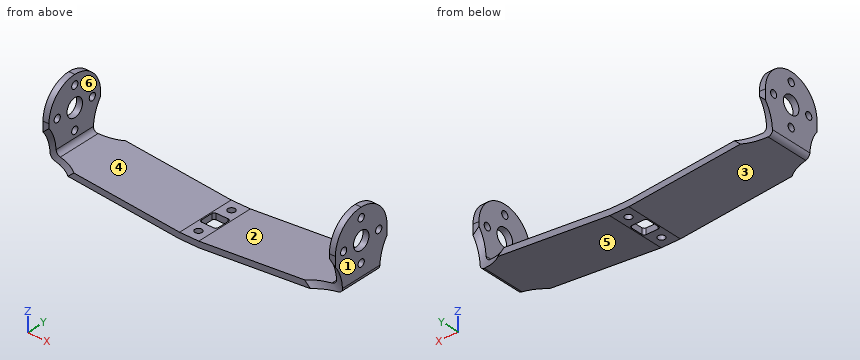
```python
from build123d import *

# Parameters (mm, degrees)
RESSALTO_EXTRUS_O1_DEPTH = 25
FILETE1_R                = 12.5
FILETE2_R                = 2
ESBO_O2_R                = 1.5
CORTE_EXTRUS_O1_DEPTH    = 10
ESBO_O3_R                = 3.75
ESBO_O3_R_2              = 1.5
CORTE_EXTRUS_O2_DEPTH    = 131.832972904
ESBO_O4_R                = 11
CORTE_EXTRUS_O5_DEPTH    = 17


with BuildPart() as part:
    # Esboço1 → Ressalto-extrusão1 (new body)
    with BuildSketch(Plane(origin=(0, 0, 0), x_dir=(1, 0, 0), z_dir=(0, 1, 0))):
        Polygon((-83.493030157, -40.103201854), (-85.993030157, -40.103201854), (-85.993030157, -12.103201854), (-28.993030157, -7.116348033), (-20.993030157, -7.116348033), (36.006969843, -12.103201854), (36.006969843, -40.103201854), (33.506969843, -40.103201854), (33.506969843, -14.394029789), (-20.993030157, -9.625897627), (-28.993030157, -9.625897627), (-83.493030157, -14.394029789), align=None)
    extrude(amount=RESSALTO_EXTRUS_O1_DEPTH)

    # Filete1
    filete1_edges = [part.edges().sort_by_distance(p)[0] for p in [
        (34.756969843, 25, 40.103201854),
        (34.756969843, 0, 40.103201854),
        (-84.743030157, 0, 40.103201854),
        (-84.743030157, 25, 40.103201854),
    ]]
    fillet(filete1_edges, radius=FILETE1_R - 0.0001)  # a hair under: the kernel refuses the full size

    # Filete2
    filete2_edges = [part.edges().sort_by_distance(p)[0] for p in [
        (-85.993030157, 12.5, 12.103201854),
        (36.006969843, 12.5, 12.103201854),
        (33.506969843, 12.5, 14.394029789),
        (-83.493030157, 12.5, 14.394029789),
    ]]
    fillet(filete2_edges, radius=FILETE2_R)

    # Esboço2 → Corte-extrusão1 (cut)
    with BuildSketch(Plane(origin=(0, 0, 7.116348033), x_dir=(-1, 0, 0), z_dir=(0, 0, -1))):
        with Locations((24.993030157, 4.5)):
            Circle(ESBO_O2_R)
        with Locations((24.993030157, 20.5)):
            Circle(ESBO_O2_R)
        with BuildLine():
            Line((27.493030157, 9), (22.493030157, 9))
            ThreePointArc((22.493030157, 9), (21.785923376, 9.292893219), (21.493030157, 10))
            Line((21.493030157, 10), (21.493030157, 15))
            ThreePointArc((21.493030157, 15), (21.785923376, 15.707106781), (22.493030157, 16))
            Line((22.493030157, 16), (27.493030157, 16))
            ThreePointArc((27.493030157, 16), (28.200136938, 15.707106781), (28.493030157, 15))
            Line((28.493030157, 15), (28.493030157, 10))
            ThreePointArc((28.493030157, 10), (28.200136938, 9.292893219), (27.493030157, 9))
        make_face()
    extrude(amount=-CORTE_EXTRUS_O1_DEPTH, mode=Mode.SUBTRACT)

    # Esboço3 → Corte-extrusão2 (cut, through all)
    with BuildSketch(Plane(origin=(36.006969843, 0, 0), x_dir=(0, 0, -1), z_dir=(1, 0, 0))):
        with Locations((-27.603201854, 12.5)):
            Circle(ESBO_O3_R)
        with Locations((-36.103201854, 12.5)):
            Circle(ESBO_O3_R_2)
        with Locations((-19.103201854, 12.5)):
            Circle(ESBO_O3_R_2)
        with Locations((-27.603201854, 4)):
            Circle(ESBO_O3_R_2)
        with Locations((-27.603201854, 21)):
            Circle(ESBO_O3_R_2)
    extrude(amount=-CORTE_EXTRUS_O2_DEPTH, mode=Mode.SUBTRACT)

    # Esboço4 → Corte-extrusão5 (cut, symmetric)
    with BuildSketch(Plane(origin=(-39.80249127, 0, -36.472263554), x_dir=(0.6755902076156622, 0, -0.7372773368101223), z_dir=(0.7372773368101223, 0, 0.6755902076156622))):
        with Locations((-67.370645943, 32.5)):
            Circle(ESBO_O4_R)
        with Locations((-67.370645943, -7.5)):
            Circle(ESBO_O4_R)
    corte_extrus_o5 = extrude(amount=CORTE_EXTRUS_O5_DEPTH, both=True, mode=Mode.SUBTRACT)

    # Espelhar1: Corte-extrusão5 across plane
    add(corte_extrus_o5.mirror(Plane(origin=(-24.993030157, 0, 0), x_dir=(0, 0, 1), z_dir=(1, 0, 0))), mode=Mode.SUBTRACT)


solid = part.part
```
Geometry: final body of the model. Coordinates: model frame, mm. Face numbers are marked on the shaded views. A direction names the side the tool comes from. Give positions to 0.01 mm unless a question says otherwise; leave off trailing zeros. Loops run counter-clockwise (first coordinate to the right, second up) from the corner with the lowest first, then second, coordinate; pieces in that order, holes last. Notation, with made-up numbers: (-37, 21) - (-17, 21) arc R21 ccw to (-17, 38) - close; hole circle Ø8 at (75.5, -28). An arc over 180 degrees is marked (long way). Answer as CSV lines item,"result". Start each with the question number.
(1) Section query A-A (x = -57). Output: boundary loops of the cut face in (y, z), and give its area (3 significant figures).
(2) Ray query, line 1 along X through (y, z) = (22, 24); line 2 along Z through (x, y) = (-25.5, 7.5); line 3 along Z through (x, y) = (27.5, 11.25). Return the intervals inside material, ascending. Write a range as [from, to].
(3) Reachability of the marked faces 5 and 6 from +Z, -Z, +X, -X, +Y, -Y: full face, straight path, thin tool, end or side. Return the list, or none.
(4) Mould query, pull axis X, two halves, no side actions, for the marked faces 1, 2, 3 and 4. Classes: +X half, -X half, draft (parallel to the pull), parting line (faces both ways), or undercut.
(5) Pin query (flat end, axial travel): P1, Ø1, axis at x = 21.5, y = 9.5, coming from the +Z side; P2, Ø9, axis at x = -25, y = 16.5, coming from the +Z side; P3, Ø4, axis at x = -60, y = 16.5, coming from the +Z side; P4, Ø4.5, axis at y = 12.5, z = 27.6, coming from the -X side. Return the tip coordinate at first contact, or that it passes through.
Worked answers:
1,outline,"(0, 9.57) - (25, 9.57) - (25, 12.08) - (0, 12.08) - close"
1,area,"62.7 mm^2"
2,line 1,"x = [-85.99, -83.49], [33.51, 36.01]"
2,line 2,"z = [7.12, 9.63]"
2,line 3,"z = [11.36, 13.87]"
3,face 5,"-Z, +X, +Y, -Y"
3,face 6,"+Z, +Y, -Y"
4,face 1,"+X half"
4,face 2,"undercut"
4,face 3,"-X half"
4,face 4,"undercut"
5,P1,"stops at z = 13.39"
5,P2,"stops at z = 9.67"
5,P3,"stops at z = 12.51"
5,P4,"passes through"
